Design review of the part built by this model. Coordinates are the model's own, in mm. A direction names the side the tool comes from. Coordinates: 2 decimals unless noted, no trailing zeros. Loops run counter-clockwise (first coordinate to the right, second up) from the corner with the lowest first, then second, coordinate; pieces in that order, holes last. Notation, with made-up numbers: (82.25, 27) - (90.25, 27) arc R36 ccw to (90.25, 66) - close; hole circle Ø10 at (10, -37.75). An arc over 180 degrees is marked (long way). Answer in a Markdown table with one row per item. Add a question column.
(1) The part is to be moulded in two halves that separate along Z. For faces 3 (the face through (-0.4, -6.6, -7)), 4 (the face through (-3, 4, -37.1)), 5 (the face through (-0.5, 0, 0)), say which applies: released by +Z, released by -Z, zero draft, split by the parting line, or undercut.
(2) Clearance check with flat-ended pins moving along their axes: pin 1 (4 mm diameter, centred on y = 5.5, z = -32, fed in from -X); pin 2 (0.6 mm diameter, centred on y = 1, z = 0, fed in from +X); pin 3 (5 mm diameter, centred on y = 2, z = -29.5, fed in from +X). State where each tip first meets the part, or that it passes through.
(3) We need section C-C, the plane x = -2.2. Write out the cut boundary in (y, z), plus the area to 3 significant figures.
(4) For faces 1 (the face through (-3.411, 4.743, -27.24)), 2 (the face through (-4.8, 6.6, -7)), list the 3-axis set-ups (+Z, -Z, +X, -X, +Y, -Y) from which the entire face can be reached by the end or side of a thin tool; tool diameter is ignored.
(5) We need section B-B, the plane z = -6.4. Write out the cut boundary in (x, y), plus the area to 3 significant figures.
(6) To check wall thickness, follow L1, parallel to Y at x = -2.4, z = -12.9; L2, parallel to Z at x = -4.8, y = -1.25; L3, parallel to X at y = -1, z = -17. State the ranges of each line that lie inside material, in increasing order. Write a range as [from, to].
(7) We need section D-D, the plane y = -4. Write out the cut boundary in (x, z), plus the area to 3 significant figures.
(8) We need section A-A, the plane y = 0. Write out the cut boundary in (x, z).
from build123d import *

# Parameters (mm, degrees)
SKETCH1_W                      = 20
SKETCH1_H                      = 14
BOSS_EXTRUDE1_DEPTH            = 5.2
SKETCH2_W                      = 1.1
SKETCH2_H                      = 10.5
CUT_EXTRUDE1_DEPTH             = 0.5
SKETCH3_W                      = 1.1
SKETCH3_H                      = 20
SKETCH4_W                      = 1.1
SKETCH4_H                      = 20
F_3_2_3_2_DIAMETER_HOLE1_D     = 3.2
F_3_2_3_2_DIAMETER_HOLE1_DEPTH = 5.2
CHAMFER1_SIZE                  = 0.8
CHAMFER2_SIZE                  = 1.4
FILLET1_R                      = 0.15
FILLET2_R                      = 0.3


with BuildPart() as part:
    # Sketch1 → Boss-Extrude1 (new body)
    with BuildSketch(Plane(origin=(0, 0, 0), x_dir=(0, 0, -1), z_dir=(1, 0, 0))):
        with Locations((7.1, 0)):
            Rectangle(SKETCH1_W, SKETCH1_H)
    extrude(amount=-BOSS_EXTRUDE1_DEPTH)

    # Sketch2 → Cut-Extrude1 (cut)
    with BuildSketch(Plane(origin=(0, 0, 0), x_dir=(0, 0, -1), z_dir=(1, 0, 0))):
        with Locations((-0.05, 0)):
            Rectangle(SKETCH2_W, SKETCH2_H)
    extrude(amount=-CUT_EXTRUDE1_DEPTH, mode=Mode.SUBTRACT)

    # Sketch3 → Revolve1 (revolve)
    with BuildSketch(Plane(origin=(0, -4, 0), x_dir=(1, 0, 0), z_dir=(0, 1, 0))):
        with Locations((-2.05, 27.1)):
            Rectangle(SKETCH3_W, SKETCH3_H)
    revolve(axis=Axis((-2.6, -4, -37.1), (0, 0, 1)))

    # Sketch4 → Revolve2 (revolve)
    with BuildSketch(Plane(origin=(0, 4, 0), x_dir=(1, 0, 0), z_dir=(0, 1, 0))):
        with Locations((-2.05, 27.1)):
            Rectangle(SKETCH4_W, SKETCH4_H)
    revolve(axis=Axis((-2.6, 4, -37.1), (0, 0, 1)))

    # Ø3.2 (3.2) Diameter Hole1
    with Locations(Plane(origin=(0, 0, 0), x_dir=(0, 0, -1), z_dir=(1, 0, 0))):
        with Locations((12.9, 0), (6.4, 0)):
            Hole(F_3_2_3_2_DIAMETER_HOLE1_D / 2, depth=F_3_2_3_2_DIAMETER_HOLE1_DEPTH)

    # Chamfer1
    chamfer1_edges = [part.edges().sort_by_distance(p)[0] for p in [
        (-5.2, 7, -7.1),
        (-5.2, -7, -7.1),
        (0, 7, -7.1),
        (0, -7, -7.1),
    ]]
    chamfer(chamfer1_edges, length=CHAMFER1_SIZE)

    # Chamfer2
    chamfer2_edges = [part.edges().sort_by_distance(p)[0] for p in [
        (0, 0, -8),
        (0, 0, -14.5),
    ]]
    chamfer(chamfer2_edges, length=CHAMFER2_SIZE)

    # Fillet1
    fillet1_edges = [part.edges().sort_by_distance(p)[0] for p in [
        (0, 0, -17.1),
        (0, 0, 2.9),
        (-2.6, 7, 2.9),
        (-5.2, 0, 2.9),
        (-2.6, -7, 2.9),
        (-4.8, 6.6, 2.9),
        (-4.8, -6.6, 2.9),
        (-0.4, -6.6, 2.9),
        (-0.4, 6.6, 2.9),
        (-2.6, 7, -17.1),
        (-2.6, -7, -17.1),
        (-5.2, 0, -17.1),
        (-4.8, 6.6, -17.1),
        (-4.8, -6.6, -17.1),
        (-0.4, -6.6, -17.1),
        (-0.4, 6.6, -17.1),
    ]]
    fillet(fillet1_edges, radius=FILLET1_R)

    # Fillet2
    fillet2_edges = [part.edges().sort_by_distance(p)[0] for p in [
        (-0.25, -5.25, -0.5),
        (-0.25, -5.25, 0.6),
        (-0.25, 5.25, 0.6),
        (-0.25, 5.25, -0.5),
    ]]
    fillet(fillet2_edges, radius=FILLET2_R)


solid = part.part
Responses:
| question | item | result |
|---|---|---|
| 1 | face 3 | zero draft |
| 1 | face 4 | released by -Z |
| 1 | face 5 | undercut |
| 2 | pin 1 | stops at x = -3.7 |
| 2 | pin 2 | stops at x = -0.5 |
| 2 | pin 3 | stops at x = -1.5 |
| 3 | outline | (-7, -16.95) arc R0.15 ccw to (-6.85, -17.1) - (-5.02, -17.1) - (-5.02, -37.1) - (-2.98, -37.1) - (-2.98, -17.1) - (2.98, -17.1) - (2.98, -37.1) - (5.02, -37.1) - (5.02, -17.1) - (6.85, -17.1) arc R0.15 ccw to (7, -16.95) - (7, 2.75) arc R0.15 ccw to (6.85, 2.9) - (-6.85, 2.9) arc R0.15 ccw to (-7, 2.75) - close; hole circle Ø3.2 at (0, -12.9); hole circle Ø3.2 at (0, -6.4) |
| 3 | area | 346 mm2 |
| 4 | face 1 | -Z |
| 4 | face 2 | +Z, -Z, -X, +Y |
| 5 | outline | (-5.2, -6.2) - (-4.4, -7) - (-0.8, -7) - (0, -6.2) - (0, -3) - (-1.4, -1.6) - (-5.2, -1.6) - close; (-5.2, 1.6) - (-1.4, 1.6) - (0, 3) - (0, 6.2) - (-0.8, 7) - (-4.4, 7) - (-5.2, 6.2) - close |
| 5 | area | 52.9 mm2 |
| 6 | L1 | y = [-7, -1.6], [1.6, 7] |
| 6 | L2 | z = [-17.1, -13.9], [-11.9, -7.4], [-5.4, 2.9] |
| 6 | L3 | x = [-5.19, -0.01] |
| 7 | outline | (-5.2, -16.95) arc R0.15 ccw to (-5.05, -17.1) - (-3.7, -17.1) - (-3.7, -37.1) - (-1.5, -37.1) - (-1.5, -17.1) - (-0.15, -17.1) arc R0.15 ccw to (0, -16.95) - (0, -0.5) - (-0.5, -0.5) - (-0.5, 0.6) - (0, 0.6) - (0, 2.75) arc R0.15 ccw to (-0.15, 2.9) - (-5.05, 2.9) arc R0.15 ccw to (-5.2, 2.75) - close |
| 7 | area | 147 mm2 |
| 8 | outline | (-5.2, -16.95) arc R0.15 ccw to (-5.05, -17.1) - (-0.15, -17.1) arc R0.15 ccw to (0, -16.95) - (0, -15.9) - (-1.4, -14.5) - (-5.2, -14.5) - close; (-5.2, -11.3) - (-1.4, -11.3) - (0, -9.9) - (0, -9.4) - (-1.4, -8) - (-5.2, -8) - close; (-5.2, -4.8) - (-1.4, -4.8) - (0, -3.4) - (0, -0.5) - (-0.5, -0.5) - (-0.5, 0.6) - (0, 0.6) - (0, 2.75) arc R0.15 ccw to (-0.15, 2.9) - (-5.05, 2.9) arc R0.15 ccw to (-5.2, 2.75) - close |
